The model under review builds one solid part; all positions refer to its coordinate system, in mm. Round coordinates to 2 decimals unless told otherwise and drop trailing zeros. Order: outer loops, then holes, each group sorted by start corner. A loop starts at its lowest first (then second) coordinate and runs counter-clockwise, first axis right, second up. Notation, with made-up numbers: M 83,-25.75 L 125,-25.75 A10 cw 125,-15.75 Z; hole C 55.5,-26 d8. An arc over 180 degrees is marked long. Answer as a JSON object with one key per item and string values. Group by question number.
1) Consider section A-A, the plane x = -42. Write out the cut boundary in (y, z).
2) To check wall thickness, follow line 1 (Z direction, x = 24.5, y = 2.3); line 2 (Z direction, x = 39, y = 3.5); line 3 (Z direction, x = -37.5, y = 3.35). State the ranges of each line that lie inside material, in increasing order.
3) Consider section D-D, the plane z = -17. Write out the cut boundary in (x, y), then the cut area to 3 significant figures.
4) Consider section C-C, the plane y = 1.45. Count the separate pieces of the cut face and the enclosed holes in it, then the cut area to 3 significant figures.
5) Consider section B-B, the plane x = 13. Write out the cut boundary in (y, z), then the cut area to 3 significant figures.
6) The part is to be moulded in two halves that separate along Z. For faces 1 (the flat face through (-1, 4.1, -1)), 2 (the flat face through (25, 2, 50)), 3 (the flat face through (0.28, 2.08, 30.83)), say which applies: +Z half, -Z half, draft (parallel to the pull), parting line (faces both ways), or undercut.
7) Insertion check: pin 1 Ø5 at (x, z) = (38.18, 38.18) entering from -Y; pin 2 Ø1.5 at (x, y) = (36, 0.5) entering from -Z; pin 3 Ø1.2 at (y, z) = (1.5, 22) entering from -X; pin 4 Ø2 at (y, z) = (1, -24) entering from +X. Each pin has a flat end and moves straight along its axis. Give the tip position at first contact, or say it passes through.
```python
from build123d import *

# Parameters (mm, degrees)
SKETCH1_W           = 100
SKETCH1_H           = 100
SKETCH1_R           = 4
SKETCH1_W_2         = 4.1
SKETCH1_H_2         = 15
SKETCH1_W_3         = 15
SKETCH1_H_3         = 4.1
BOSS_EXTRUDE1_DEPTH = 4.1
CUT_EXTRUDE1_START  = 35
SKETCH2_W           = 141.421356238
SKETCH2_H           = 4.1
CUT_EXTRUDE1_DEPTH  = 35.710678
CUT_EXTRUDE2_REACH  = 107.711
CUT_EXTRUDE2_START  = -35
SKETCH3_W           = 141.421356238
SKETCH3_H           = 4.1
CUT_EXTRUDE3_DEPTH  = 5.1


with BuildPart() as part:
    # Sketch1 → Boss-Extrude1 (new body)
    with BuildSketch(Plane(origin=(0, 0, 0), x_dir=(1, 0, 0), z_dir=(0, 1, 0))):
        Rectangle(SKETCH1_W, SKETCH1_H)
        with Locations((38.183766184, -38.183766184)):
            Circle(SKETCH1_R, mode=Mode.SUBTRACT)
        with Locations((-22.95, 37.5)):
            Rectangle(SKETCH1_W_2, SKETCH1_H_2, mode=Mode.SUBTRACT)
        with Locations((-37.5, 22.95)):
            Rectangle(SKETCH1_W_3, SKETCH1_H_3, mode=Mode.SUBTRACT)
        with Locations((37.5, -22.95)):
            Rectangle(SKETCH1_W_3, SKETCH1_H_3, mode=Mode.SUBTRACT)
        with Locations((22.95, -37.5)):
            Rectangle(SKETCH1_W_2, SKETCH1_H_2, mode=Mode.SUBTRACT)
        with Locations((37.5, 22.95)):
            Rectangle(SKETCH1_W_3, SKETCH1_H_3, mode=Mode.SUBTRACT)
        with Locations((-37.5, -22.95)):
            Rectangle(SKETCH1_W_3, SKETCH1_H_3, mode=Mode.SUBTRACT)
        with Locations((22.95, 37.5)):
            Rectangle(SKETCH1_W_2, SKETCH1_H_2, mode=Mode.SUBTRACT)
        with Locations((-22.95, -37.5)):
            Rectangle(SKETCH1_W_2, SKETCH1_H_2, mode=Mode.SUBTRACT)
    extrude(amount=BOSS_EXTRUDE1_DEPTH)

    # Sketch2 → Cut-Extrude1 (cut)
    with BuildSketch(Plane(origin=(0, 0, 0), x_dir=(0.707106781, 0, 0.707106781), z_dir=(-0.707106781, 0, 0.707106781)).offset(CUT_EXTRUDE1_START)):
        with Locations((0, 2.05)):
            Rectangle(SKETCH2_W, SKETCH2_H)
    extrude(amount=CUT_EXTRUDE1_DEPTH, mode=Mode.SUBTRACT)

    # Sketch3 → Cut-Extrude2 (cut, up to next)
    with BuildSketch(Plane(origin=(0, 0, 0), x_dir=(0.707106781, 0, 0.707106781), z_dir=(-0.707106781, 0, 0.707106781)).offset(CUT_EXTRUDE2_START), mode=Mode.PRIVATE) as cut_extrude2_sk1:
        with Locations((0, 2.05)):
            Rectangle(SKETCH3_W, SKETCH3_H)
    cut_extrude2_tool1 = extrude(cut_extrude2_sk1.sketch, amount=-CUT_EXTRUDE2_REACH, mode=Mode.PRIVATE) & part.part
    add(cut_extrude2_tool1.solids().sort_by_distance((24.748737, 2.05, -24.748737))[0], mode=Mode.SUBTRACT)

    # Sketch4 → Cut-Extrude3 (cut, through all)
    with BuildSketch(Plane(origin=(0, 4.1, 0), x_dir=(1, 0, 0), z_dir=(0, 1, 0))):
        Polygon((-38.961583643, -2.050609665), (-36.062445841, -4.949747468), (-25.455844123, 5.656854249), (-28.354981926, 8.555992052), align=None)
        Polygon((8.555992052, -28.354981926), (-2.050609665, -38.961583643), (-4.949747468, -36.062445841), (5.656854249, -25.455844123), align=None)
        Polygon((38.961583643, 2.050609665), (36.062445841, 4.949747468), (25.455844123, -5.656854249), (28.354981926, -8.555992052), align=None)
        Polygon((-8.555992052, 28.354981926), (2.050609665, 38.961583643), (4.949747468, 36.062445841), (-5.656854249, 25.455844123), align=None)
    extrude(amount=-CUT_EXTRUDE3_DEPTH, mode=Mode.SUBTRACT)


solid = part.part
```
Results list:
{
 "1": {"outline": "M 0,-50 L 4.1,-50 L 4.1,-25 L 0,-25 Z; M 0,-20.9 L 4.1,-20.9 L 4.1,7.5 L 0,7.5 Z"},
 "2": {"line 1": "-25 to 30, 45 to 50", "line 2": "-10.5 to 20.9, 25 to 34.27, 42.1 to 50", "line 3": "-50 to -25, -20.9 to 0.59, 3.51 to 12"},
 "3": {"outline": "M -50,0 L 32.5,0 L 32.5,4.1 L -50,4.1 Z", "area": "338 mm^2"},
 "4": {"separate pieces": "1", "enclosed holes": "9", "area": "6,910 mm^2"},
 "5": {"outline": "M 0,-36.5 L 4.1,-36.5 L 4.1,50 L 0,50 Z", "area": "355 mm^2"},
 "6": {"face 1": "draft", "face 2": "+Z half", "face 3": "undercut"},
 "7": {"pin 1": "through", "pin 2": "z = -14.25", "pin 3": "x = -28.1", "pin 4": "x = 26.5"}
}
